The listing builds one solid part. Answer for the finished solid, in the listing's coordinates (mm). Round coordinates to 2 decimals unless told otherwise and drop trailing zeros. Order: outer loops, then holes, each group sorted by start corner. A loop starts at its lowest first (then second) coordinate and runs counter-clockwise, first axis right, second up. Notation, with made-up numbers: (55.25, 45.5) -> (92.25, 45.5) arc R25 cw to (92.25, 61.5) -> close; hole circle Ø2 at (18, 37.5). An arc over 180 degrees is marked (long way). Answer in a Markdown table with one row per item. Add a question column.
Autodesk Inventor part; units mm, degrees
ref_plane "YZ Plane" through (0, 0, 0) normal (1, 0, 0) x (0, 1, 0)
ref_plane "XZ Plane" through (0, 0, 0) normal (0, 1, 0) x (-1, 0, 0)
ref_plane "XY Plane" through (0, 0, 0) normal (0, 0, 1) x (1, 0, 0)
sketch "Sketch1" plane through (0, 0, 0) normal (1, 0, 0) x (0, 1, 0)
  circle A0 centre (0, 0) radius 2.5
  arc A1 (-4.0201, -2) -> (-4.0201, 2) centre (0, 0) ccw
  line L0 (0, 0) -> (-177.8, 0) construction
  circle A2 centre (-177.8, 0) radius 2.5
  arc A3 (-173.1955, 2) -> (-173.1955, -2) centre (-177.8, 0) ccw
  line L1 (-4.0201, 2) -> (-173.1955, 2)
  line L2 (-4.0201, -2) -> (-173.1955, -2)
  dimension "d0" = 5
  dimension "d1" = 1.9901
  dimension "d2" = 177.8
  dimension "d3" = 5
  dimension "d4" = 2.5201
  dimension "d9" = 4
  dimension "d10" = 2
extrude "Extrusion1" add sketch "Sketch1" along normal blind 4
chamfer "Chamfer1" distance 1.6 angle 45 8 edges at (4, -88.6078, 2) (0, -88.6078, 2) (0, -88.6078, -2) (4, -88.6078, -2) (0, 4.4901, 0) (4, 4.4901, 0) (0, -182.8201, 0) (4, -182.8201, 0)
sketch "Sketch2" plane through (0, 0, 0) normal (0, 0, 1) x (1, 0, 0)
  line L0 (4, 2.5) -> (4, -2.5)
  line L1 (0, 2.5) -> (0, -2.5)
  line L2 (4, -175.3) -> (4, -180.3)
  line L3 (0, -175.3) -> (0, -180.3)
  line L4 (4, 2.5) -> (4, -2.5) construction
  line L5 (4, 0) -> (0, 0)
  line L6 (0, 2.5) -> (0, -2.5) construction
  line L7 (0, -175.3) -> (0, -180.3) construction
  line L8 (0, -177.8) -> (4, -177.8) construction
  line L9 (4, -175.3) -> (4, -180.3) construction
  circle A0 centre (2, 0) radius 3
  circle A1 centre (2, -177.8) radius 3
  line L10 (-1, -177.8) -> (5, -177.8)
  line L11 (5, 0) -> (-1, 0)
  dimension "d14" = 6
  dimension "d15" = 6
revolve "Revolution1" cut sketch "Sketch2" angle 360 about axis through (-1, -177.8, 0) along (1, 0, 0) picked at (4.1409, -179.1351) picked at (2, -178.8) picked at (-0.1409, -179.1351) contours L10 A1 L2 | L2 A1 L3 L10 | L3 A1 L10
sketch "Sketch3" plane through (0, 0, 0) normal (0, 0, 1) x (1, 0, 0)
  line L0 (4, 2.5) -> (4, -2.5)
  line L1 (0, 2.5) -> (0, -2.5)
  line L2 (4, -175.3) -> (4, -180.3)
  line L3 (0, -175.3) -> (0, -180.3)
  line L4 (4, 2.5) -> (4, -2.5) construction
  line L5 (4, 0) -> (0, 0)
  line L6 (0, 2.5) -> (0, -2.5) construction
  line L7 (0, -175.3) -> (0, -180.3) construction
  line L8 (0, -177.8) -> (4, -177.8) construction
  line L9 (4, -175.3) -> (4, -180.3) construction
  circle A0 centre (2, 0) radius 3
  circle A1 centre (2, -177.8) radius 3
  line L10 (-1, -177.8) -> (5, -177.8)
  line L11 (5, 0) -> (-1, 0)
  dimension "d17" = 6
  dimension "d18" = 6
revolve "Revolution2" cut sketch "Sketch3" angle 360 about axis through (5, 0, 0) along (-1, 0, 0) picked at (4.1409, 1.3351) picked at (2, 1) picked at (-0.1409, 1.3351) contours A0 L11 L0 | L0 L5 L1 A0 | L1 L11 A0
properties part number "Delta Robot Arm Segment Two"
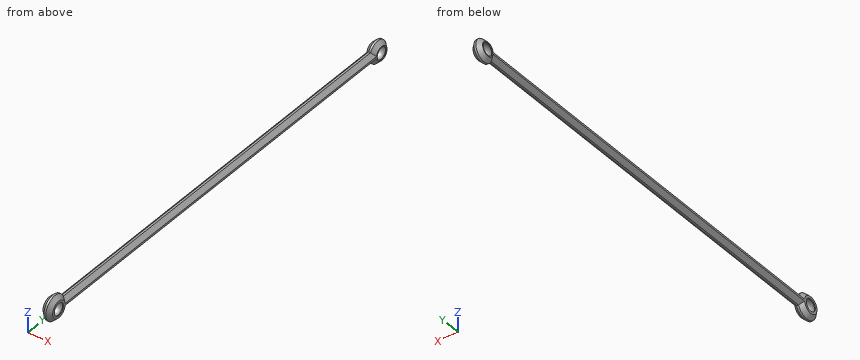
Item 1: Find the intervals of material crossed by probe 1 along Y at (x, z) = (2.4, 0); probe 2 along Y at (x, z) = (1.4, 0.25); probe 3 along Z at (x, y) = (2.25, -79.5), in increasing order. Write a range as [from, to].
Item 2: The part is cut by section B-B, the plane y = -61.5. Give the vertices of the cut face in (x, z).
Item 3: The part is cut by section A-A, the plane y = -177.8. Give the vertices of the cut face in (x, z), and give its area (3 significant figures).
Item 4: Flat-ended cylindrical pins translate along their axes: P1, Ø1, axis at x = 0.5, y = -79, coming from the +Z side; P2, Ø4.5, axis at y = -177.8, z = 0, coming from the -X side; P3, Ø1, axis at y = -65.5, z = 2, coming from the -X side; P4, Ø1, axis at x = 2, y = -136.5, coming from the +Z side. Find the tip coordinate at first contact, or state that the pin passes through.
Item 5: The part is cut by section C-C, the plane y = 0. Give the vertices of the cut face in (x, z), and give its area (3 significant figures).
Resolved:
| question | item | result |
|---|---|---|
| 1 | probe 1 | [-182.82, -180.77], [-174.83, -2.97], [2.97, 4.49] |
| 1 | probe 2 | [-182.61, -180.73], [-174.87, -2.93], [2.93, 4.28] |
| 1 | probe 3 | [-2, 2] |
| 2 | outline | (0, -0.4) -> (1.6, -2) -> (2.4, -2) -> (4, -0.4) -> (4, 0.4) -> (2.4, 2) -> (1.6, 2) -> (0, 0.4) -> close |
| 3 | outline | (0, -3.42) -> (1.6, -5.02) -> (2.4, -5.02) -> (4, -3.42) -> (4, -2.5) -> (3.66, -2.5) arc R3 cw to (0.34, -2.5) -> (0, -2.5) -> close; (0, 2.5) -> (0.34, 2.5) arc R3 cw to (3.66, 2.5) -> (4, 2.5) -> (4, 3.42) -> (2.4, 5.02) -> (1.6, 5.02) -> (0, 3.42) -> close |
| 3 | area | 12.8 mm2 |
| 4 | P1 | z = 1.4 |
| 4 | P2 | through |
| 4 | P3 | x = 1.1 |
| 4 | P4 | z = 2 |
| 5 | outline | (0, -2.89) -> (1.6, -4.49) -> (2.4, -4.49) -> (4, -2.89) -> (4, -2.5) -> (3.66, -2.5) arc R3 cw to (0.34, -2.5) -> (0, -2.5) -> close; (0, 2.5) -> (0.34, 2.5) arc R3 cw to (3.66, 2.5) -> (4, 2.5) -> (4, 2.89) -> (2.4, 4.49) -> (1.6, 4.49) -> (0, 2.89) -> close |
| 5 | area | 8.55 mm2 |
